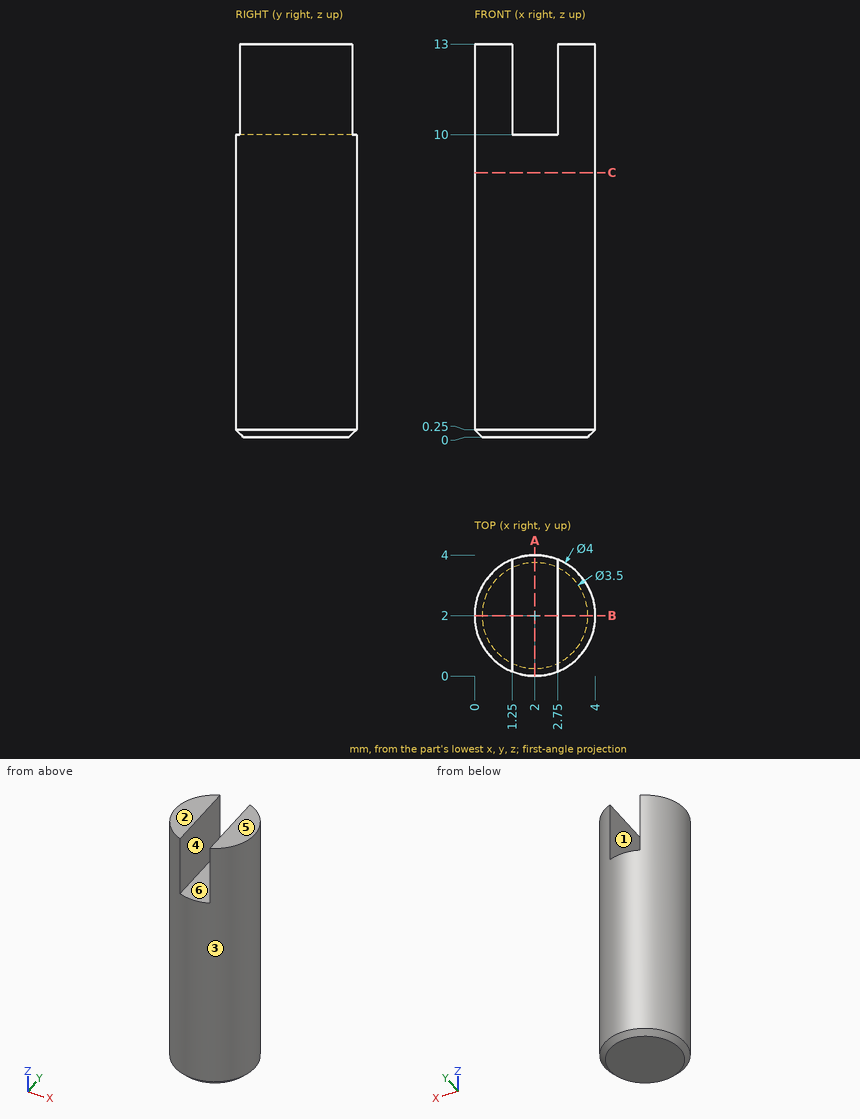
Input: dimensioned drawing with shaded views. Units: mm. Origin: part minimum x, y, z. A direction names the side the tool comes from. Give positions to 0.01 mm unless a question says otherwise; leave off trailing zeros. Write each loop counter-clockwise with the first axis right and the second up, starting at its lowest first coordinate (ties: lowest second). Pieces come first, ordered by that corner, then holes. Notation, with made-up numbers: (-2.75, -11) -> (4.25, -11) arc R27 cw to (4.25, 14) -> close; hole circle Ø4 at (15, 83.25). An arc over 180 degrees is marked (long way). Return JSON: item names as keys, results as strings. Group by question number.
1. Section B-B, the plane y = 2. Output: boundary loops of the cut face in (x, z), then the cut area to 3 significant figures.
2. Access query for the marked faces 1 and 2. Directions: +Z, -Z, +X, -X, +Y, -Y. A direction counts if a zero-diameter tool reaches every point of the face in a straight line with its end or side. Return the directions, or none.
3. Section A-A, the plane x = 2. Output: boundary loops of the cut face in (y, z).
4. Mould query, pull axis X, two halves, no side actions, for the marked faces 3, 4, 5 and 6. Classes: +X half, -X half, draft (parallel to the pull), parting line (faces both ways), or undercut.
5. Section C-C, the plane z = 8.75. Output: boundary loops of the cut face in (x, y).
6. Material intervals for line 1 (Y direction, x = 2.1, z = 7); line 2 (Z direction, x = 1.65, y = 3.55); line 3 (Y direction, x = 1.25, z = 6), sorted ascending. Write a range as from..to.
Determined:
{
 "1": {"outline": "(0, 0.25) -> (0.25, 0) -> (3.75, 0) -> (4, 0.25) -> (4, 13) -> (2.75, 13) -> (2.75, 10) -> (1.25, 10) -> (1.25, 13) -> (0, 13) -> close", "area": "47.4 mm2"},
 "2": {"face 1": "+Z, +Y, -Y", "face 2": "+Z, +X, -X, +Y, -Y"},
 "3": {"outline": "(0, 0.25) -> (0.25, 0) -> (3.75, 0) -> (4, 0.25) -> (4, 10) -> (0, 10) -> close"},
 "4": {"face 3": "parting line", "face 4": "undercut", "face 5": "draft", "face 6": "undercut"},
 "5": {"outline": "circle Ø4 at (2, 2)"},
 "6": {"line 1": "y = 0..4", "line 2": "z = 0..10", "line 3": "y = 0.15..3.85"}
}
